Read the model definition and answer for the solid it produces. Units are mm, in the model's axes. Coordinates: 2 decimals unless noted, no trailing zeros. Order: outer loops, then holes, each group sorted by start corner. A loop starts at its lowest first (then second) coordinate and runs counter-clockwise, first axis right, second up. Notation, with made-up numbers: M 7,51.25 L 23,51.25 A22 cw 23,89.25 Z; hole C 76,-14.5 d4. An arc over 180 degrees is marked long. Use a Markdown table: item, result. Add a question column.
1) Find section D-D on z = 8. Write down the section's boundary in (x, y), plus the area to 3 significant figures.
2) Find section B-B on z = 0. Write down the section's boundary in (x, y).
3) Find section A-A on x = 0. Write down the section's boundary in (y, z).
4) Each of these flat-tipped pins is pushed along its axis until it touches: pin 1 Ø3.5 at (x, z) = (-21.21, -21.21) entering from +Y; pin 2 Ø2 at (x, y) = (0, 5.5) entering from +Z; pin 3 Ø3 at (y, z) = (5.5, -1.5) entering from +X; pin 4 Ø3 at (y, z) = (4.5, 0) entering from -X. Where does it stop, or does it pass through?
5) Find section C-C on y = 6. Count the separate pieces of the cut face and the enclosed holes in it, plus the area to 3 significant figures.
6) Find the intervals of material crossed by probe 1 along Z at (x, y) = (0, 1); probe 2 along X at (y, z) = (1.75, -0.5); probe 3 along Z at (x, y) = (2, 2), in increasing order. Write a range as [from, to].
from build123d import *

# Parameters (mm, degrees)
SKETCH1_R                    = 36
SKETCH1_R_2                  = 22
BOSS_EXTRUDE1_DEPTH          = 3
BOSS_EXTRUDE2_DEPTH          = 6
SKETCH3_R                    = 2.5
BOSS_EXTRUDE3_DEPTH          = 5
CHAMFER1_SIZE                = 1.2
CIRPATTERN1_COUNT            = 4
CHAMFER1_OF_CIRPATTERN1_SIZE = 1.2
SKETCH4_R                    = 1.6
CUT_EXTRUDE1_DEPTH           = 3
CIRPATTERN2_COUNT            = 4


with BuildPart() as part:
    # Sketch1 → Boss-Extrude1 (new body)
    with BuildSketch(Plane(origin=(0, 0, 0), x_dir=(1, 0, 0), z_dir=(0, 1, 0))):
        Circle(SKETCH1_R)
        Circle(SKETCH1_R_2, mode=Mode.SUBTRACT)
    extrude(amount=BOSS_EXTRUDE1_DEPTH)

    # Sketch2 → Boss-Extrude2 (add)
    with BuildSketch(Plane(origin=(0, 3, 0), x_dir=(1, 0, 0), z_dir=(0, 1, 0))):
        with BuildLine():
            Line((-32.829457155, 3.5), (-35.829457155, 3.5))
            ThreePointArc((-35.829457155, 3.5), (-36, 0), (-35.829457155, -3.5))
            Line((-35.829457155, -3.5), (-32.829457155, -3.5))
            Line((-32.829457155, -3.5), (-32.829457155, 3.5))
        make_face()
    boss_extrude2 = extrude(amount=BOSS_EXTRUDE2_DEPTH)

    # Sketch3 → Boss-Extrude3 (add)
    with BuildSketch(Plane(origin=(-32.829457155, 0, 0), x_dir=(0, 0, -1), z_dir=(1, 0, 0))):
        with Locations((0, 6)):
            Circle(SKETCH3_R)
    boss_extrude3 = extrude(amount=BOSS_EXTRUDE3_DEPTH)

    # Chamfer1
    chamfer1_edges = [part.edges().sort_by_distance(p)[0] for p in [
        (-27.829457155, 6, 2.5),
    ]]
    chamfer(chamfer1_edges, length=CHAMFER1_SIZE)

    # CirPattern1: Boss-Extrude2, Boss-Extrude3 ×4 about axis
    cirpattern1_axis = Axis((0, 0, 0), (0, 1, 0))
    for i in range(1, CIRPATTERN1_COUNT):
        add(boss_extrude2.rotate(cirpattern1_axis, i * 360 / CIRPATTERN1_COUNT))
        add(boss_extrude3.rotate(cirpattern1_axis, i * 360 / CIRPATTERN1_COUNT))

    # Chamfer1 of CirPattern1
    chamfer1_of_cirpattern1_edges = [part.edges().sort_by_distance(p)[0] for p in [
        (2.5, 6, 27.829457155),
        (27.829457155, 6, -2.5),
        (-2.5, 6, -27.829457155),
    ]]
    chamfer(chamfer1_of_cirpattern1_edges, length=CHAMFER1_OF_CIRPATTERN1_SIZE)

    # Sketch4 → Cut-Extrude1 (cut)
    with BuildSketch(Plane(origin=(0, 3, 0), x_dir=(1, 0, 0), z_dir=(0, 1, 0))):
        with Locations((-21.213203436, 21.213203436)):
            Circle(SKETCH4_R)
    cut_extrude1 = extrude(amount=-CUT_EXTRUDE1_DEPTH, mode=Mode.SUBTRACT)

    # CirPattern2: Cut-Extrude1 ×4 about axis
    cirpattern2_axis = Axis((0, 0, 0), (0, 1, 0))
    for i in range(1, CIRPATTERN2_COUNT):
        add(cut_extrude1.rotate(cirpattern2_axis, i * 360 / CIRPATTERN2_COUNT), mode=Mode.SUBTRACT)


solid = part.part
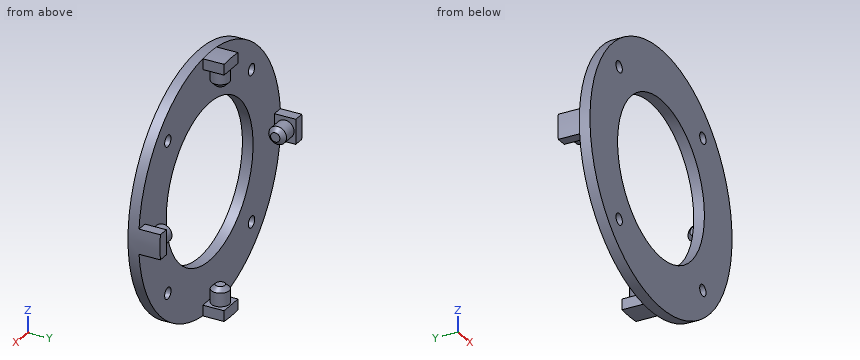
Check result:
| question | item | result |
|---|---|---|
| 1 | outline | M -35.1,0 L -20.49,0 L -20.49,3 L -35.1,3 Z; M 20.49,0 L 35.1,0 L 35.1,3 L 20.49,3 Z |
| 1 | area | 87.6 mm2 |
| 2 | outline | M -36,0 L -22,0 L -22,3 L -32.83,3 L -32.83,3.5 L -29.03,3.5 L -27.83,4.7 L -27.83,7.3 L -29.03,8.5 L -32.83,8.5 L -32.83,9 L -36,9 Z; M 22,0 L 36,0 L 36,9 L 32.83,9 L 32.83,8.5 L 29.03,8.5 L 27.83,7.3 L 27.83,4.7 L 29.03,3.5 L 32.83,3.5 L 32.83,3 L 22,3 Z |
| 3 | outline | M 0,-36 L 9,-36 L 9,-32.83 L 8.5,-32.83 L 8.5,-29.03 L 7.3,-27.83 L 4.7,-27.83 L 3.5,-29.03 L 3.5,-32.83 L 3,-32.83 L 3,-22 L 0,-22 Z; M 0,22 L 3,22 L 3,32.83 L 3.5,32.83 L 3.5,29.03 L 4.7,27.83 L 7.3,27.83 L 8.5,29.03 L 8.5,32.83 L 9,32.83 L 9,36 L 0,36 Z |
| 4 | pin 1 | stops at y = 3 |
| 4 | pin 2 | stops at z = 36 |
| 4 | pin 3 | stops at x = 36 |
| 4 | pin 4 | stops at x = -36 |
| 5 | separate pieces | 4 |
| 5 | enclosed holes | 0 |
| 5 | area | 181 mm2 |
| 6 | probe 1 | z = [-36, -22], [22, 36] |
| 6 | probe 2 | x = [-36, -21.99], [21.99, 36] |
| 6 | probe 3 | z = [-35.94, -21.91], [21.91, 35.94] |
